The listing builds one solid part. Answer for the finished solid, in the listing's coordinates (mm). A direction names the side the tool comes from. Give positions to 0.01 mm unless a question says otherwise; leave off trailing zeros. Write each loop counter-clockwise with the first axis right and the second up, starting at its lowest first coordinate (ties: lowest second). Pieces come first, ordered by that corner, then holes. Notation, with made-up numbers: M 82,-39 L 120,-39 A7 cw 120,-29 Z; hole C 14.25,22.5 d10. An arc over 180 degrees is marked long. Return JSON: item names as keys, results as strings.
from build123d import *

# Parameters (mm, degrees)
BASE_FLANGE2_DEPTH             = 1
EDGE_FLANGE1_STRIP_W           = 6
EDGE_FLANGE1_STRIP_H           = 1
EDGE_FLANGE1_STRIP_CUT_DEPTH   = 82.6
EDGE_FLANGE1_STRIP_2_W         = 6
EDGE_FLANGE1_STRIP_2_H         = 1
EDGE_FLANGE1_STRIP_CUT_2_DEPTH = 82.6
EDGE_FLANGE1_DEPTH             = 82.6
EDGE_FLANGE1_BEND_DEPTH        = 82.6
SKETCH16_W                     = 66.6
SKETCH16_H                     = 7
CUT_EXTRUDE1_DEPTH             = 138.553195479
FILLET1_R                      = 1
SKETCH17_R                     = 2
CUT_EXTRUDE2_DEPTH             = 138.553195479
CUT_EXTRUDE3_DEPTH             = 138.553195479
FILLET2_R                      = 2.5


# Sheet-metal steps are written as plain solids
with BuildPart() as part:
    # Sketch1 → Base-Flange2 (new body)
    with BuildSketch(Plane(origin=(0, 0, 0), x_dir=(1, 0, 0), z_dir=(0, 1, 0))):
        Polygon((0, 0), (0, 82.6), (5, 82.6), (12.071067812, 89.671067812), (92.000932188, 89.671067812), (99.072, 82.6), (104.072, 82.6), (104.072, 0), (99.072, 0), (92.000932188, -7.071067812), (12.071067812, -7.071067812), (5, 0), align=None)
    extrude(amount=-BASE_FLANGE2_DEPTH)

    # Edge-Flange1 strip (across the edge) → Edge-Flange1 strip cut (cut)
    with BuildSketch(Plane(origin=(104.072, 0, 0), x_dir=(-1, 0, 0), z_dir=(0, 0, -1))):
        with Locations((-1, -0.5)):
            Rectangle(EDGE_FLANGE1_STRIP_W, EDGE_FLANGE1_STRIP_H)
    extrude(amount=EDGE_FLANGE1_STRIP_CUT_DEPTH, mode=Mode.SUBTRACT)

    # Edge-Flange1 strip 2 (across the edge) → Edge-Flange1 strip cut 2 (cut)
    with BuildSketch(Plane.XY.offset(-82.6)):
        with Locations((-1, -0.5)):
            Rectangle(EDGE_FLANGE1_STRIP_2_W, EDGE_FLANGE1_STRIP_2_H)
    extrude(amount=EDGE_FLANGE1_STRIP_CUT_2_DEPTH, mode=Mode.SUBTRACT)

    # Edge-Flange1 section (across the edge) → Edge-Flange1 (add)
    with BuildSketch(Plane(origin=(104.072, 0, 0), x_dir=(-1, 0, 0), z_dir=(0, 0, -1))):
        with BuildLine():
            Line((0, 1), (0, 7))
            Line((0, 7), (1, 7))
            Line((1, 7), (1, 1))
            ThreePointArc((1, 1), (1.292893219, 0.292893219), (2, 0))
            Line((2, 0), (2, -1))
            ThreePointArc((2, -1), (0.585786438, -0.414213562), (0, 1))
        make_face()
    extrude(amount=EDGE_FLANGE1_DEPTH)

    # Edge-Flange1 section 2 (across the edge) → Edge-Flange1 bend (add)
    with BuildSketch(Plane.XY.offset(-82.6)):
        with BuildLine():
            Line((0, 1), (0, 7))
            Line((0, 7), (1, 7))
            Line((1, 7), (1, 1))
            ThreePointArc((1, 1), (1.292893219, 0.292893219), (2, 0))
            Line((2, 0), (2, -1))
            ThreePointArc((2, -1), (0.585786438, -0.414213562), (0, 1))
        make_face()
    extrude(amount=EDGE_FLANGE1_BEND_DEPTH)

    # Sketch16 → Cut-Extrude1 (cut, through all)
    with BuildSketch(Plane(origin=(104.072, 0, 0), x_dir=(0, 0, -1), z_dir=(1, 0, 0))):
        with Locations((41.3, 4.5)):
            Rectangle(SKETCH16_W, SKETCH16_H)
    extrude(amount=-CUT_EXTRUDE1_DEPTH, mode=Mode.SUBTRACT)

    # Fillet1
    fillet1_edges = [part.edges().sort_by_distance(p)[0] for p in [
        (0.5, 7, -74.6),
        (0.5, 7, -8),
        (103.572, 7, -8),
        (103.572, 7, -74.6),
        (103.572, 7, 0),
        (103.572, 7, -82.6),
        (0.5, 7, -82.6),
        (0.5, 7, 0),
    ]]
    fillet(fillet1_edges, radius=FILLET1_R)

    # Sketch17 → Cut-Extrude2 (cut, through all)
    with BuildSketch(Plane(origin=(104.072, 0, 0), x_dir=(0, 0, -1), z_dir=(1, 0, 0))):
        with Locations(Location((4, 4, 0), (0, 0, 90))):
            Circle(SKETCH17_R)
        with Locations(Location((78.6, 4, 0), (0, 0, 90))):
            Circle(SKETCH17_R)
    extrude(amount=-CUT_EXTRUDE2_DEPTH, mode=Mode.SUBTRACT)

    # Sketch19 → Cut-Extrude3 (cut, through all)
    with BuildSketch(Plane(origin=(0, 0, 0), x_dir=(1, 0, 0), z_dir=(0, 1, 0))):
        Polygon((15, -2.071067812), (83.072, -2.071067812), (83.072, 7.928932188), (97.072, 7.928932188), (97.072, 74.671067812), (83.072, 74.671067812), (83.072, 84.671067812), (15, 84.671067812), (15, 77.671067812), (7, 77.671067812), (7, 4.928932188), (15, 4.928932188), align=None)
    extrude(amount=-CUT_EXTRUDE3_DEPTH, mode=Mode.SUBTRACT)

    # Fillet2
    fillet2_edges = [part.edges().sort_by_distance(p)[0] for p in [
        (12.071067812, -0.5, -89.671067812),
        (92.000932188, -0.5, -89.671067812),
        (92.000932188, -0.5, 7.071067812),
        (12.071067812, -0.5, 7.071067812),
        (15, -0.5, 2.071067812),
        (15, -0.5, -4.928932188),
        (7, -0.5, -4.928932188),
        (7, -0.5, -77.671067812),
        (15, -0.5, -77.671067812),
        (15, -0.5, -84.671067812),
        (83.072, -0.5, -84.671067812),
        (83.072, -0.5, -74.671067812),
        (97.072, -0.5, -74.671067812),
        (97.072, -0.5, -7.928932188),
        (83.072, -0.5, -7.928932188),
        (83.072, -0.5, 2.071067812),
    ]]
    fillet(fillet2_edges, radius=FILLET2_R)


solid = part.part
Item 1: Determine the mould class of faces 1 (the cylindrical face through (0.507, 3.566, -80.552)), 2 (the cylindrical face through (96.36, -0.51, -8.68)), 3 (the flat face through (1, 6, -5)), 4 (the flat face through (95.947, -0.493, 3.125)) for opening direction Z: +Z half, -Z half, draft (parallel to the pull), parting line (faces both ways), or undercut.
Geometry results:
{"face 1": "undercut", "face 2": "undercut", "face 3": "draft", "face 4": "+Z half"}
Item 2: Which of the six approach directions +Z, -Z, +X, -X, +Y, -Y give full straight-line access (tool end or side, diameter ignored) to faces 5 (the flat face through (0.8, 1.5, -82.6)), 6 (the flat face through (8.2, -0.5, 3.2)), 7 (the cylindrical face through (96.32, -0.51, -73.96)), 8 (the flat face through (100, 0, -42))?
Geometry results:
{"face 5": "-Z, -X, +Y, -Y", "face 6": "+Z, -X, +Y, -Y", "face 7": "+Y, -Y", "face 8": "+Z, -Z, +Y"}
Item 3: A cutting plane is placed at A-A, the plane x = 22. Write down the section's boundary in (y, z), plus the area to 3 significant figures.
Geometry results:
{"outline": "M -1,-89.67 L 0,-89.67 L 0,-84.67 L -1,-84.67 Z; M -1,2.07 L 0,2.07 L 0,7.07 L -1,7.07 Z", "area": "10.0 mm2"}
Item 4: Find the intervals of material crossed by line 1 (Z direction, x = 103.35, y = 4); line 2 (Z direction, x = 80, y = -0.5); line 3 (X direction, y = 0.75, z = -10), in increasing order.
Geometry results:
{"line 1": "z = -82.6 to -80.6, -76.6 to -74.6, -8 to -6, -2 to 0", "line 2": "z = -89.67 to -84.67, 2.07 to 7.07", "line 3": "x = 0.02 to 1.03, 103.04 to 104.06"}
Item 5: A cutting plane is placed at B-B, the plane y = 4. Count the separate pieces of the cut face and the enclosed holes in it, plus the area to 3 significant figures.
Geometry results:
{"separate pieces": "8", "enclosed holes": "0", "area": "16.0 mm2"}
Item 6: Given pin 1 Ø0.8 at (y, z) = (-0.5, -78.5) entering from -X; pin 2 Ø4 at (x, y) = (2.5, 2.5) entering from -Z; pin 3 Ø0.5 at (x, y) = (103.5, 3.5) entering from +Z, each flat-ended and moving along its own axis, determine where each tip first touches the part or whether it passes through.
Geometry results:
{"pin 1": "stops at x = 0.33", "pin 2": "stops at z = -82.6", "pin 3": "stops at z = 0"}
Item 7: A cutting plane is placed at C-C, the plane z = -22.5. Write down the section's boundary in (x, y), plus the area to 3 significant figures.
Geometry results:
{"outline": "M 0,1 A2 ccw 2,-1 L 7,-1 L 7,0 L 2,0 A1 cw 1,1 Z; M 97.07,-1 L 102.07,-1 A2 ccw 104.07,1 L 103.07,1 A1 cw 102.07,0 L 97.07,0 Z", "area": "14.7 mm2"}
